Input: part model. Units: mm. Frame: model coordinates. Coordinates: 2 decimals unless noted, no trailing zeros. Write each loop counter-clockwise with the first axis right and the second up, starting at its lowest first coordinate (ties: lowest second). Pieces come first, ordered by that corner, then holes. Notation, with made-up numbers: (-19.5, 68.5) - (-15.5, 68.5) arc R32 cw to (-15.5, 96.5) - close; hole circle Ø1 at (4.5, 26.25). An arc over 180 degrees is marked (long way). One line per question, with ' | ' between items. Start each with the question number.
1) Line query: line 1 (Y direction, x = 13.5, z = 2) (3 decimals); line 2 (X direction, y = 2.25, z = 1); line 3 (X direction, y = 3.5, z = 6.25). Output: solid intervals per line, ascending.
2) Draft query along X for faces 1 (the cylindrical face through (11.342, 3.27, 3.131)), 2 (the cylindrical face through (4.88, 4.75, 3.13)), 3 (the flat face through (0, 3, 3)), 4 (the flat face through (13, 6.35, 3)). Return one class per face: released by +X, released by -X, zero draft, split by the parting line, or undercut.
3) Section query B-B on y = 2.5. Return loops of the section in (x, z).
4) Section query D-D on z = 3.5. Give the number of separate pieces and of enclosed holes in the cut face, and give its area (3 significant figures).
5) Section query A-A on x = 13.5. Return loops of the section in (y, z) (3 decimals).
6) Section query C-C on y = 1.25. Return loops of the section in (x, z), and give its area (3 significant figures).
```python
from build123d import *

# Parameters (mm, degrees)
SKETCH1_W           = 27
SKETCH1_H           = 6.35
SKETCH1_R           = 2.16
SKETCH1_R_2         = 1.5875
BOSS_EXTRUDE1_DEPTH = 6.35
CHAMFER1_SIZE       = 0.5


with BuildPart() as part:
    # Sketch1 → Boss-Extrude1 (new body)
    with BuildSketch(Plane.XY):
        with Locations((13.5, 3.175)):
            Rectangle(SKETCH1_W, SKETCH1_H)
        with Locations((13.5, 3.175)):
            Circle(SKETCH1_R, mode=Mode.SUBTRACT)
        with Locations((5.0875, 3.175)):
            Circle(SKETCH1_R_2, mode=Mode.SUBTRACT)
    extrude(amount=BOSS_EXTRUDE1_DEPTH)

    # Chamfer1
    chamfer1_edges = [part.edges().sort_by_distance(p)[0] for p in [
        (0, 6.35, 3.175),
        (27, 6.35, 3.175),
        (27, 0, 3.175),
        (0, 0, 3.175),
    ]]
    chamfer(chamfer1_edges, length=CHAMFER1_SIZE)


solid = part.part
```
Answer key:
1) line 1: 0 to 1.015, 5.335 to 6.35 | line 2: 0 to 3.8, 6.38 to 11.55, 15.45 to 27 | line 3: 0 to 3.53, 6.64 to 11.36, 15.64 to 27
2) face 1: undercut | face 2: undercut | face 3: released by -X | face 4: zero draft
3) outline: (0, 0) - (3.65, 0) - (3.65, 6.35) - (0, 6.35) - close; (6.52, 0) - (11.45, 0) - (11.45, 6.35) - (6.52, 6.35) - close; (15.55, 0) - (27, 0) - (27, 6.35) - (15.55, 6.35) - close
4) separate pieces: 1 | enclosed holes: 2 | area: 148 mm²
5) outline: (0, 0) - (1.015, 0) - (1.015, 6.35) - (0, 6.35) - close; (5.335, 0) - (6.35, 0) - (6.35, 6.35) - (5.335, 6.35) - close
6) outline: (0, 0) - (12.52, 0) - (12.52, 6.35) - (0, 6.35) - close; (14.48, 0) - (27, 0) - (27, 6.35) - (14.48, 6.35) - close | area: 159 mm²
